The model under review builds one solid part; all positions refer to its coordinate system, in mm. Face numbers are marked on the shaded views. A direction names the side the tool comes from. Coordinates: 2 decimals unless noted, no trailing zeros. Write each loop counter-clockwise with the first axis right and the second up, starting at its lowest first coordinate (ties: lowest second). Pieces come first, ordered by that corner, then holes.
1) For P1, Ø3.5, axis at x = -25.22, y = -4.1, coming from the +Z side; P2, Ø1.5, axis at x = -30, y = -24.5, coming from the +Z side, all flat-tipped, find the tip position at first contact; note any pin that passes through.
2) Add section C-C, the plane z = 9.75. State the section outline as (x, y) points, then the cut area to 3 significant figures.
3) Add section D-D, the plane x = -56. State the section outline as (y, z) points.
4) Add section A-A, the plane x = -42.5. State the section outline as (y, z) points, then the cut area to 3 significant figures.
5) Add section B-B, the plane y = -1. State the section outline as (x, z) points.
6) Mouldability with a two-part tool opening along X and no side actions: class the marked faces 1, 2 and 3 as released by +X, released by -X, zero draft, split by the parting line, or undercut.
7) For line 1 (Y direction, x = -37, z = 15.25); line 2 (X direction, y = -14, z = 18); line 3 (Z direction, x = -61, y = 3), list the stretches that pass through material, from the lowest coordinate up.
8) Machinability: for the marked faces 4 and 5, which of the approach directions +Z, -Z, +X, -X, +Y, -Y give a long, thin tool a straight path to every point of the face, cutting with its end or side? Answer none if there is none.
from build123d import *

# Parameters (mm, degrees)
F0_W     = 45
F0_H     = 45
F1_DEPTH = 2
F2_W     = 45
F2_H     = 45
F2_W_2   = 41
F2_H_2   = 41
F3_DEPTH = 20
F4_W     = 8
F4_H     = 2
F5_DEPTH = 2
F6_R     = 2
F7_DEPTH = 25


with BuildPart() as f1:
    # F0 (on Top) → F1 (new body)
    with BuildSketch(Plane.XY):
        with Locations((-42.720676, -16.595085)):
            Rectangle(F0_W, F0_H)
    extrude(amount=F1_DEPTH)

    # F2 (on face) → F3 (join)
    with BuildSketch(Plane.XY.offset(2)):
        with Locations((-42.720676, -16.595085)):
            Rectangle(F2_W, F2_H)
        with Locations((-42.720676, -16.595085)):
            Rectangle(F2_W_2, F2_H_2, mode=Mode.SUBTRACT)
    extrude(amount=F3_DEPTH)

    # F4 (on face) → F5 (cut, through all)
    with BuildSketch(Plane(origin=(0, 0, 0), x_dir=(1, 0, 0), z_dir=(0, 0, -1))):
        with Locations((-42.720676, 1.095085)):
            Rectangle(F4_W, F4_H)
    extrude(amount=-F5_DEPTH, mode=Mode.SUBTRACT)

    # F6 (on face) → F7 (cut)
    with BuildSketch(Plane(origin=(0, 0, 0), x_dir=(1, 0, 0), z_dir=(0, 0, -1))):
        with Locations((-25.220676, 4.095085)):
            Circle(F6_R)
        with Locations((-60.220676, 4.095085)):
            Circle(F6_R)
    extrude(amount=-F7_DEPTH, mode=Mode.SUBTRACT)


solid = f1.part
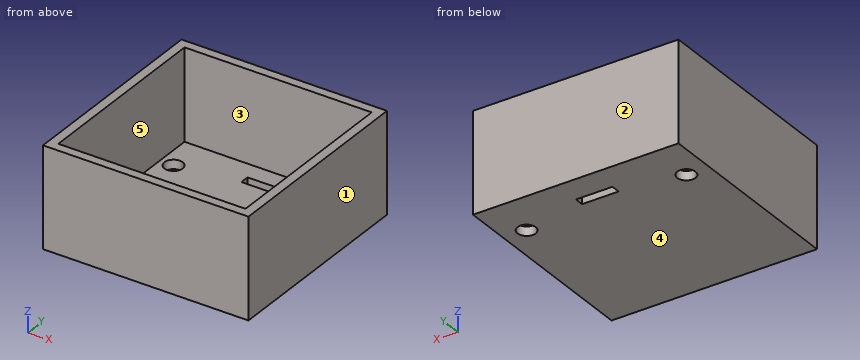
Geometry results:
1. P1: passes through
1. P2: stops at z = 2
2. outline: (-65.22, -39.1) - (-20.22, -39.1) - (-20.22, 5.9) - (-65.22, 5.9) - close; hole (-63.22, -37.1) - (-22.22, -37.1) - (-22.22, 3.9) - (-63.22, 3.9) - close
2. area: 344 mm2
3. outline: (-39.1, 0) - (5.9, 0) - (5.9, 22) - (3.9, 22) - (3.9, 2) - (-37.1, 2) - (-37.1, 22) - (-39.1, 22) - close
4. outline: (-39.1, 0) - (-2.1, 0) - (-2.1, 2) - (-37.1, 2) - (-37.1, 22) - (-39.1, 22) - close; (-0.1, 0) - (5.9, 0) - (5.9, 22) - (3.9, 22) - (3.9, 2) - (-0.1, 2) - close
4. area: 166 mm2
5. outline: (-65.22, 0) - (-46.72, 0) - (-46.72, 2) - (-63.22, 2) - (-63.22, 22) - (-65.22, 22) - close; (-38.72, 0) - (-20.22, 0) - (-20.22, 22) - (-22.22, 22) - (-22.22, 2) - (-38.72, 2) - close
6. face 1: released by +X
6. face 2: zero draft
6. face 3: undercut
7. line 1: y = -39.1 to -37.1, 3.9 to 5.9
7. line 2: x = -65.22 to -63.22, -22.22 to -20.22
7. line 3: z = 0 to 2
8. face 4: -Z, +X, -X, +Y, -Y
8. face 5: +Z
